Autodesk Inventor part; units mm, degrees
ref_plane "Начальная плоскость" through (0, 0, -22.5) normal (0, 0, 1) x (1, 0, 0)
ref_plane "Конечная плоскость" through (0, 0, 1822.5) normal (0, 0, 1) x (1, 0, 0)
ref_plane "РабПлоскость4" through (-1.43, 0, 1822.5) normal (0.7071, 0, 0.7071) x (0.7071, 0, -0.7071)
ref_plane "Начальная плоскость" through (0, 0, -22.5) normal (0, 0, 1) x (1, 0, 0)
ref_plane "Конечная плоскость" through (0, 0, 1822.5) normal (0, 0, 1) x (1, 0, 0)
sketch "Эскиз" plane through (0, 0, 0) normal (0, 0, 1) x (1, 0, 0)
  line L0 (-1.43, 0) -> (-1.43, 40)
  line L1 (-1.43, 40) -> (43.57, 40)
  line L2 (43.57, 40) -> (43.57, 38.1774)
  line L3 (39.9881, 34.1993) -> (11.2338, 31.1771)
  line L4 (4.07, 23.221) -> (4.07, 0)
  line L5 (4.07, 0) -> (-1.43, 0) construction
  line L6 (23.82, 40) -> (23.82, 32.5) construction
  line L7 (43.57, 34.5758) -> (43.57, 32.5) construction
  line L8 (43.57, 32.5) -> (23.82, 32.5) construction
  line L9 (0, 15) -> (0, -27) construction
  line L10 (-5.539, 0) -> (16.0067, 0) construction
  line L11 (-1.43, 0) -> (-1.43, -40)
  line L12 (-1.43, -40) -> (43.57, -40)
  line L13 (43.57, -40) -> (43.57, -38.1774)
  line L14 (39.9881, -34.1993) -> (11.2338, -31.1771)
  line L15 (4.07, -23.221) -> (4.07, 0)
  arc A0 (11.2338, 31.1771) -> (4.07, 23.221) centre (12.07, 23.221) ccw
  arc A1 (4.07, -23.221) -> (11.2338, -31.1771) centre (12.07, -23.221) ccw
  arc A2 (39.9881, 34.1993) -> (43.57, 38.1774) centre (39.57, 38.1774) ccw
  arc A3 (43.57, -38.1774) -> (39.9881, -34.1993) centre (39.57, -38.1774) ccw
  line L16 (0, 56) -> (0, -56) construction
  line L17 (-15.5135, 0) -> (54.308, 0) construction
  point P0 (4.07, 30.4242)
  point P1 (43.57, -34.5758)
  point P2 (4.07, -30.4242)
  point P3 (23.82, -40)
  point P4 (23.82, -32.5)
  dimension "d0" = 5.5
  dimension "d1" = 40
  dimension "d2" = 45
  dimension "d3" = 7.5
  dimension "d4" = 19.75
  dimension "d5" = 2.0758
  dimension "d23" = 8
  dimension "d24" = 4
  dimension "d25" = 1.43
extrude "Тело" add sketch "Эскиз" along normal up to surface (1845 mm away) from surface at -22.5
sketch "Sketch3" plane through (0, 0, 0) normal (0, 0, 1) x (1, 0, 0)
  line L0 (0, 0) -> (10, 0)
ref_plane "Work Plane3" through (0, 0, 0) normal (0, -1, 0) x (1, 0, 0)
sketch "Sketch4" plane through (0, 0, 0) normal (0, -1, 0) x (1, 0, 0)
  line L0 (-2, -22.5) -> (12, -22.5)
  line L1 (-2, 1822.5) -> (12, 1822.5)
  dimension "d29" = 1845
ref_plane "РабПлоскость4" through (-1.43, 0, 1822.5) normal (0.7071, 0, 0.7071) x (0.7071, 0, -0.7071)
split "Разделение1" plane through (-1.43, 0, 1822.5) removes the side toward (0.7071, 0, 0.7071)
ref_plane "РабПлоскость5" through (-1.43, 0, -22.5) normal (0.7071, 0, -0.7071) x (-0.7071, 0, -0.7071)
split "Разделение2" plane through (-1.43, 0, -22.5) removes the side toward (0.7071, 0, -0.7071)
equation "\"d0\" = G_T"
equation "\"d1\" = 0.5 * G_H"
equation "\"d2\" = G_W"
equation "\"d3\" = G_T1"
equation "\"d4\" = G_C"
equation "\"d23\" = G_IR"
equation "\"d24\" = G_ER"
equation "\"d25\" = ex"
equation "\"d6\" = G_L"
equation "\"G_W\" = 45"
equation "\"G_T\" = 5.5"
equation "\"G_T1\" = 7.5"
equation "\"G_NG\" = 0.105104"
equation "\"G_ER\" = 4"
equation "\"G_IR\" = 8"
equation "\"G_C\" = 19.75"
equation "\"G_L\" = d29"
equation "\"ex\" = 1.43"
equation "\"G_OFFSET_START\" = 22.5"
equation "\"G_OFFSET_END\" = 22.5"
equation "\"d26\" = -G_OFFSET_START"
equation "\"d27\" = G_OFFSET_END + B_L"
properties part number "ISO 657/11 - CH 80 x 8 - 1845" material "Сталь нержавеющая, 440C"
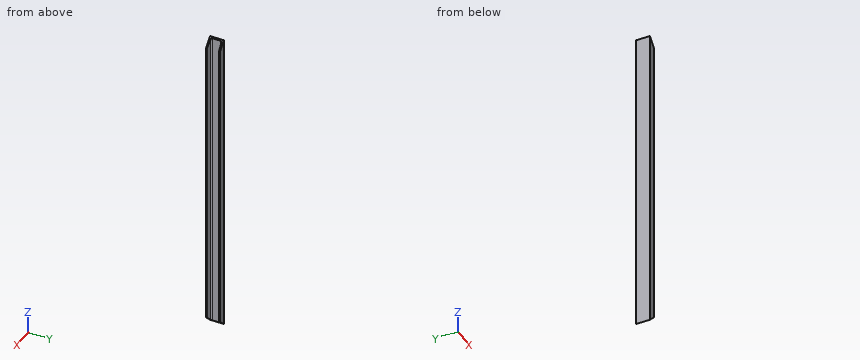
Geometry: final body of the model. Coordinates: model frame, mm. Round coordinates to 2 decimals unless told otherwise and drop trailing zeros. Write each loop counter-clockwise with the first axis right and the second up, starting at its lowest first coordinate (ties: lowest second). Pieces come first, ordered by that corner, then holes. Notation, with made-up numbers: M 12,80.25 L 30,80.25 A10 cw 30,91.25 Z; hole C 36,77 d2. An arc over 180 degrees is marked long. Answer in a Markdown table with one row per item. Add a question column.
(1) Ray query, L1, parallel to Y at x = 13, z = 814; L2, parallel to Y at x = 37.5, z = 1355.5; L3, parallel to X at y = -17, z = 304.5. Return the intervals inside material, ascending.
(2) Contact query for flat-ended pins moving along their axis: pin 1 (5 mm diameter, centred on x = 4, y = -23, fed in from -Z); pin 2 (12 mm diameter, centred on y = 5.5, z = 1046.5, fed in from +X). Output: stop coordinate, or through.
(3) Cut plane A-A, the plane x = 31.5. Return the cut outline in (y, z).
(4) Cut plane B-B, the plane z = 387. Return the cut outline in (x, y).
(5) Cut plane C-C, the plane y = 7. Return the cut outline in (x, z), then the cut area to 3 significant figures.
Established:
| question | item | result |
|---|---|---|
| 1 | L1 | -40 to -31.36, 31.36 to 40 |
| 1 | L2 | -40 to -33.94, 33.94 to 40 |
| 1 | L3 | -1.43 to 4.07 |
| 2 | pin 1 | z = -19.57 |
| 2 | pin 2 | x = 4.07 |
| 3 | outline | M -40,10.43 L -33.31,10.43 L -33.31,1789.57 L -40,1789.57 Z; M 33.31,10.43 L 40,10.43 L 40,1789.57 L 33.31,1789.57 Z |
| 4 | outline | M -1.43,-40 L 43.57,-40 L 43.57,-38.18 A4 ccw 39.99,-34.2 L 11.23,-31.18 A8 cw 4.07,-23.22 L 4.07,23.22 A8 cw 11.23,31.18 L 39.99,34.2 A4 ccw 43.57,38.18 L 43.57,40 L -1.43,40 Z |
| 5 | outline | M -1.43,-22.5 L 4.07,-17 L 4.07,1817 L -1.43,1822.5 Z |
| 5 | area | 10,100 mm² |
